Read the model definition and answer for the solid it produces. Units are mm, in the model's axes. Face numbers are marked on the shaded views. A direction names the side the tool comes from. Give positions to 0.01 mm unless a question says otherwise; leave off trailing zeros. Loops run counter-clockwise (first coordinate to the right, second up) from the corner with the lowest first, then second, coordinate; pieces in that order, holes last. Notation, with made-up numbers: (68.5, 53.5) - (78.5, 53.5) arc R31 cw to (78.5, 84.5) - close; hole circle Ø4 at (81, 77.25). An arc over 180 degrees is marked (long way). Put each result on its own line as item: value. Start each with the question number.
1. For the marked faces 1 and 2, determine the directions among +Z, -Z, +X, -X, +Y, -Y from which every point of the face is accessible in a straight line to the end or side of a thin tool.
2. A cutting plane is placed at C-C, the plane z = 10.25. Determine the outline of the cut face in (x, y), plus the area to 3 significant figures.
3. A cutting plane is placed at A-A, the plane x = 6. Determine the outline of the cut face in (y, z), plus the area to 3 significant figures.
4. Given pin 1 Ø4 at (y, z) = (-3, 14.5) entering from -X, flat-ended and moving along its own axis, determine where the tip first touches the part or whether it passes through.
5. A cutting plane is placed at D-D, the plane x = 12. Determine the outline of the cut face in (y, z).
6. Consider L1, parallel to Z at x = -0.5, y = -11; L2, parallel to Z at x = 13, y = -12; L3, parallel to X at y = -1, z = 14.25. Determine where each line is inside the solid, lowest interval first. Write a range as from..to.
7. A cutting plane is placed at B-B, the plane y = -12. Determine the outline of the cut face in (x, z).
```python
from build123d import *

# Parameters (mm, degrees)
F1_DEPTH = 15
F2_R     = 5
F3_R     = 2


with BuildPart() as f1:
    # F0 (on Front) → F1 (new body)
    with BuildSketch(Plane.XZ):
        with BuildLine():
            Line((-20, 5), (-25, 0))
            Line((-25, 0), (20, 0))
            Line((20, 0), (20, 20.5))
            Line((20, 20.5), (-25, 20.5))
            Line((-25, 20.5), (-20, 15.5))
            Line((-20, 15.5), (8.997297, 15.5))
            ThreePointArc((8.997297, 15.5), (14.247297, 10.25), (8.997297, 5))
            Line((8.997297, 5), (-20, 5))
        make_face()
    extrude(amount=F1_DEPTH)

    # F2
    f2_edges = [f1.edges().sort_by_distance(p)[0] for p in [
        (20, -7.5, 20.5),
        (20, -7.5, 0),
    ]]
    fillet(f2_edges, radius=F2_R)

    # F3
    f3_edges = [f1.edges().sort_by_distance(p)[0] for p in [
        (-25, -7.5, 20.5),
        (-20, -7.5, 5),
        (-25, -7.5, 0),
        (-20, -7.5, 15.5),
    ]]
    fillet(f3_edges, radius=F3_R)


solid = f1.part
```
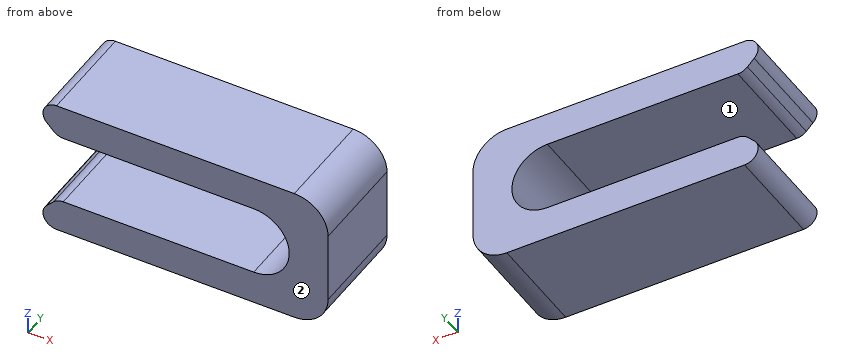
Return value:
1. face 1: -X, +Y, -Y
1. face 2: +Z, -Z, +X, -X, -Y
2. outline: (14.25, -15) - (20, -15) - (20, 0) - (14.25, 0) - close
2. area: 86.3 mm2
3. outline: (-15, 0) - (0, 0) - (0, 5) - (-15, 5) - close; (-15, 15.5) - (0, 15.5) - (0, 20.5) - (-15, 20.5) - close
3. area: 150 mm2
4. pin 1: stops at x = -21
5. outline: (-15, 0) - (0, 0) - (0, 5.94) - (-15, 5.94) - close; (-15, 14.56) - (0, 14.56) - (0, 20.5) - (-15, 20.5) - close
6. L1: z = 0..5, 15.5..20.5
6. L2: z = 0..6.85, 13.65..20.5
6. L3: x = 12.4..20
7. outline: (-21.59, 3.41) arc R2 ccw to (-20.17, 0) - (15, 0) arc R5 ccw to (20, 5) - (20, 15.5) arc R5 ccw to (15, 20.5) - (-20.17, 20.5) arc R2 ccw to (-21.59, 17.09) - (-20.59, 16.09) arc R2 ccw to (-19.17, 15.5) - (9, 15.5) arc R5.25 cw to (9, 5) - (-19.17, 5) arc R2 ccw to (-20.59, 4.41) - close
